```python
from build123d import *

# Parameters (mm, degrees)
F0_R     = 14.5
F1_DEPTH = 19
F2_R     = 6.8
F3_DEPTH = 6
F4_W     = 10.5
F4_H     = 10.5
F5_DEPTH = 10


# Not quite as in the source:
# - a feature of the source that left no trace in its solid (it failed there, or was rolled back) is left out


with BuildPart() as f1:
    # F0 (on Top) → F1 (new body)
    with BuildSketch(Plane.XY):
        Circle(F0_R)
    extrude(amount=F1_DEPTH)

    # F2 (on face) → F3 (join)
    with BuildSketch(Plane.XY.offset(19)):
        Circle(F2_R)
    extrude(amount=F3_DEPTH)

    # F4 (on face) → F5 (cut)
    with BuildSketch(Plane(origin=(0, 0, 0), x_dir=(1, 0, 0), z_dir=(0, 0, -1))):
        Rectangle(F4_W, F4_H)
    extrude(amount=-F5_DEPTH, mode=Mode.SUBTRACT)


solid = f1.part
```
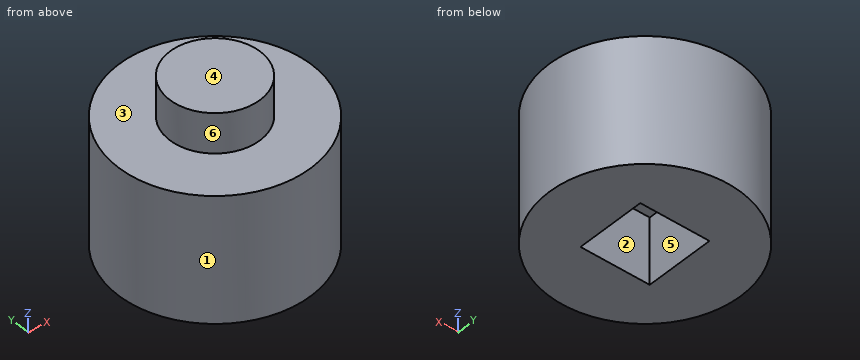
For this review, take the finished solid that the model builds, in its own axes (mm). Face numbers are marked on the shaded views. A direction names the side the tool comes from. Round coordinates to 2 decimals unless told otherwise and drop trailing zeros. Order: outer loops, then holes, each group sorted by start corner. A loop starts at its lowest first (then second) coordinate and runs counter-clockwise, first axis right, second up.
Q1. Insertion check: P1, Ø3, axis at x = -5.5, y = 11, coming from the +Z side; P2, Ø2, axis at y = 5.5, z = 20.5, coming from the -X side; P3, Ø5, axis at x = 6.5, z = 22, coming from the +Y side. Each pin has a flat end and moves straight along its axis. Give the tip position at first contact, or say it passes through.
Findings below:
P1: stops at z = 19
P2: stops at x = -5.1
P3: stops at y = 5.5
Q2. Machinability: for the marked faces 1, 2 and 3, which of the approach directions +Z, -Z, +X, -X, +Y, -Y give a long, thin tool a straight path to every point of the face, cutting with its end or side? Answer none if there is none.
Findings below:
face 1: +Z, -Z
face 2: -Z
face 3: +Z
Q3. We need section A-A, the plane z = 6.75. Give the boundary of the cut face in (x, y).
Findings below:
outline: circle Ø29 at (0, 0); hole (-5.25, -5.25) - (5.25, -5.25) - (5.25, 5.25) - (-5.25, 5.25) - close
Q4. Mouldability with a two-part tool opening along X and no side actions: class the marked faces 4, 5 and 6 as pulls with the +X half, pulls with the -X half, needs draft (parallel to the pull), parting line crosses it, or undercut.
Findings below:
face 4: needs draft
face 5: undercut
face 6: parting line crosses it
Q5. We need section D-D, the plane z = 19.5. Give the boundary of the cut face in (x, y).
Findings below:
outline: circle Ø13.6 at (0, 0)
Q6. Wall thickness on line 1 (Z direction, x = -11.25, y = -0.5); line 2 (Z direction, x = -2.5, y = 1); line 3 (X direction, y = -0.25, z = 20.5): over which ranges is each line inside the solid? List them lowest first.
Findings below:
line 1: z = 0 to 19
line 2: z = 10 to 25
line 3: x = -6.8 to 6.8
Q7. We need section B-B, the plane y = 0. Give the boundary of the cut face in (x, z), plus the area to 3 significant figures.
Findings below:
outline: (-14.5, 0) - (-5.25, 0) - (-5.25, 10) - (5.25, 10) - (5.25, 0) - (14.5, 0) - (14.5, 19) - (6.8, 19) - (6.8, 25) - (-6.8, 25) - (-6.8, 19) - (-14.5, 19) - close
area: 528 mm2
